```python
from build123d import *

# Parameters (mm, degrees)
F1_DEPTH  = 9.03
F2_W      = 29
F2_H      = 2.03
F3_DEPTH  = 25.001
F4_W      = 15
F4_H      = 29
F5_DEPTH  = 3
F7_DEPTH  = 3
F8_R      = 1.55
F9_DEPTH  = 3
F10_R     = 4
F11_DEPTH = 9.031


with BuildPart() as f1:
    # F0 (on Top) → F1 (new body)
    with BuildSketch(Plane.XY):
        with BuildLine():
            ThreePointArc((15.4117660597, 18.6968654121), (2.9117660597, 31.1968654121), (-9.5882339403, 18.6968654121))
            Line((-9.5882339403, 18.6968654121), (15.4117660597, 18.6968654121))
        make_face()
        with BuildLine():
            Line((15.4117660597, 18.6968654121), (-9.5882339403, 18.6968654121))
            ThreePointArc((-9.5882339403, 18.6968654121), (2.9117660597, 6.1968654121), (15.4117660597, 18.6968654121))
        make_face()
        with BuildLine():
            ThreePointArc((15.4117660597, 18.6968654121), (2.9117660597, 6.1968654121), (-9.5882339403, 18.6968654121))
            Line((-9.5882339403, 18.6968654121), (-9.5882339403, -14.3031345879))
            Line((-9.5882339403, -14.3031345879), (15.4117660597, -14.3031345879))
            Line((15.4117660597, -14.3031345879), (15.4117660597, 18.6968654121))
        make_face()
    extrude(amount=F1_DEPTH)

    # F2 (on face) → F3 (cut, through all)
    with BuildSketch(Plane(origin=(-9.5882339403, 0, 0), x_dir=(0, -1, 0), z_dir=(-1, 0, 0))):
        with Locations((-2.1968654121, 5.015)):
            Rectangle(F2_W, F2_H)
    extrude(amount=-F3_DEPTH, mode=Mode.SUBTRACT)

    # F4 (on face) → F5 (cut, through all)
    with BuildSketch(Plane.XY.offset(9.03)):
        with Locations((2.9117660597, 2.1968654121)):
            Rectangle(F4_W, F4_H)
    extrude(amount=-F5_DEPTH, mode=Mode.SUBTRACT)

    # F6 (on face) → F7 (join)
    with BuildSketch(Plane.XY.offset(9.03)):
        Polygon((2.9117660597, -2.9356375903), (-4.5882339403, -12.3031345879), (10.4117660597, -12.3031345879), align=None)
        Polygon((10.4117660597, 16.6968654121), (-4.5882339403, 16.6968654121), (2.9117660597, 7.3293684145), align=None)
    extrude(amount=-F7_DEPTH)

    # F8 (on face) → F9 (cut, through all)
    with BuildSketch(Plane.XY.offset(9.03)):
        with Locations((12.9117660597, 2.1968654121)):
            Circle(F8_R)
    extrude(amount=-F9_DEPTH, mode=Mode.SUBTRACT)

    # F10 (on face) → F11 (cut, through all)
    with BuildSketch(Plane.XY.offset(9.03)):
        with Locations((2.9117660597, 25.1968654121)):
            Circle(F10_R)
    extrude(amount=-F11_DEPTH, mode=Mode.SUBTRACT)


solid = f1.part
```
Here's how the part is built. I have some questions about the finished solid (model axes, mm). A direction names the side the tool comes from. Coordinates: 2 decimals unless noted, no trailing zeros. Order: outer loops, then holes, each group sorted by start corner. A loop starts at its lowest first (then second) coordinate and runs counter-clockwise, first axis right, second up. Notation, with made-up numbers: (22.5, -21) - (81.5, -21) arc R16 cw to (81.5, -17) - close; hole circle Ø1 at (71.25, -27.75). An arc over 180 degrees is marked (long way). One line per question, with ' | ' between items. Start each with the question number.
1. Please list where these lines run through material, in increasing order: line 1 along X through (y, z) = (-4.5, 6.75); line 2 along X through (y, z) = (-9, 6.75); line 3 along Z through (x, y) = (13.25, 7). Write a range as [from, to].
2. If we section it at D-D (y = 3): Write out the boundary of the cut face in (x, z), and give its area (3 significant figures).
3. I'm going to push flat-ended pins straight in: pin 1 Ø2 at (x, z) = (5.5, 5) entering from +Y; pin 2 Ø5 at (x, z) = (-6, 1.5) entering from +Y; pin 3 Ø0.6 at (x, z) = (3.5, 4.5) entering from +Y. Where does each tip first touch, or does it pass through?
4. If we section it at C-C (x = 2.25): Write out the boundary of the cut face in (y, z), and give its area (3 significant figures).
5. If we section it at A-A (y = -2): Write out the boundary of the cut face in (x, z), and give its area (3 significant figures).
6. Which directions (+Z, -Z, +X, -X, +Y, -Y) give clear straight access to the entire face, cutting with the end or side of a thin tool? Please do faces 1 (the flat face through (3, 9, 9.03)), 2 (the flat face through (3, 16.697, 5)), 3 (the flat face through (6.61, 11.95, 7.55)).
7. If we mould it in two halves opening along X, with no side actions, what happens to faces 4 (the flat face through (6.71, -7.68, 7.55)), 5 (the flat face through (3, 13, 6.03)), 6 (the cylindrical face through (3.187, 31.194, 4.452))? For each: released by +X, released by -X, zero draft, split by the parting line, or undercut.
8. If we section it at B-B (z = 5.5): Write out the boundary of the cut face in (x, y), and give its area (3 significant figures).
Model answer:
1) line 1: x = [-9.59, -4.59], [1.66, 4.16], [10.41, 15.41] | line 2: x = [-9.59, -4.59], [-1.94, 7.77], [10.41, 15.41] | line 3: z = [0, 4], [6.03, 9.03]
2) outline: (-9.59, 0) - (15.41, 0) - (15.41, 4) - (-9.59, 4) - close; (-9.59, 6.03) - (-4.59, 6.03) - (-4.59, 9.03) - (-9.59, 9.03) - close; (10.41, 6.03) - (11.59, 6.03) - (11.59, 9.03) - (10.41, 9.03) - close; (14.24, 6.03) - (15.41, 6.03) - (15.41, 9.03) - (14.24, 9.03) - close | area: 122 mm²
3) pin 1: stops at y = 31.1 | pin 2: stops at y = 29.43 | pin 3: stops at y = 31.19
4) outline: (-14.3, 0) - (21.25, 0) - (21.25, 9.03) - (8.16, 9.03) - (8.16, 6.03) - (16.7, 6.03) - (16.7, 4) - (-12.3, 4) - (-12.3, 6.03) - (-3.76, 6.03) - (-3.76, 9.03) - (-14.3, 9.03) - close; (29.14, 0) - (31.18, 0) - (31.18, 9.03) - (29.14, 9.03) - close | area: 245 mm²
5) outline: (-9.59, 0) - (15.41, 0) - (15.41, 4) - (-9.59, 4) - close; (-9.59, 6.03) - (-4.59, 6.03) - (-4.59, 9.03) - (-9.59, 9.03) - close; (10.41, 6.03) - (15.41, 6.03) - (15.41, 9.03) - (10.41, 9.03) - close | area: 130 mm²
6) face 1: +Z, +X, -X, +Y, -Y | face 2: +X, -X | face 3: +Z
7) face 4: undercut | face 5: zero draft | face 6: split by the parting line
8) outline: (-9.59, -14.3) - (15.41, -14.3) - (15.41, -12.3) - (-9.59, -12.3) - close; (-9.59, 16.7) - (15.41, 16.7) - (15.41, 18.7) arc R12.5 ccw to (-9.59, 18.7) - close; hole circle Ø8 at (2.91, 25.2) | area: 295 mm²
